from build123d import *

# Parameters (mm, degrees)
SKETCH_1_R          = 5.6
EXTRUDE_1_DEPTH     = 10
SKETCH_9_R          = 2.5
CUT_EXTRUDE_1_DEPTH = 6
SKETCH_11_R         = 2.5
CUT_EXTRUDE_2_DEPTH = 12


with BuildPart() as part:
    # 草图1 → 凸台-拉伸1 (new body)
    with BuildSketch(Plane.XY):
        with BuildLine():
            Line((-9.061643836, 9.77739726), (6.938356164, 9.77739726))
            ThreePointArc((6.938356164, 9.77739726), (8.352569727, 9.191610823), (8.938356164, 7.77739726))
            Line((8.938356164, 7.77739726), (8.938356164, -17.22260274))
            Line((8.938356164, -17.22260274), (-11.061643836, -17.22260274))
            Line((-11.061643836, -17.22260274), (-11.061643836, 7.77739726))
            ThreePointArc((-11.061643836, 7.77739726), (-10.475857398, 9.191610823), (-9.061643836, 9.77739726))
        make_face()
        with Locations((-1.061643836, -0.22260274)):
            Circle(SKETCH_1_R, mode=Mode.SUBTRACT)
    extrude(amount=EXTRUDE_1_DEPTH)

    # 草图9 → 切除-拉伸1 (cut)
    with BuildSketch(Plane(origin=(0, 9.77739726, 0), x_dir=(1, 0, 0), z_dir=(0, 1, 0))):
        with Locations((-1.061643836, -5)):
            Circle(SKETCH_9_R)
    extrude(amount=-CUT_EXTRUDE_1_DEPTH, mode=Mode.SUBTRACT)

    # 草图11 → 切除-拉伸2 (cut)
    with BuildSketch(Plane.XZ.offset(17.22260274)):
        with Locations((-6.061643836, 5)):
            Circle(SKETCH_11_R)
        with Locations((3.938356164, 5)):
            Circle(SKETCH_11_R)
    extrude(amount=-CUT_EXTRUDE_2_DEPTH, mode=Mode.SUBTRACT)


solid = part.part
CAD build for the part. Positions are in the model's coordinates, mm. A direction names the side the tool comes from. Round coordinates to 2 decimals unless told otherwise and drop trailing zeros. Write each loop counter-clockwise with the first axis right and the second up, starting at its lowest first coordinate (ties: lowest second). Pieces come first, ordered by that corner, then holes. Notation, with made-up numbers: (56, 23) -> (85, 23) arc R15 cw to (85, 35) -> close; hole circle Ø6 at (77, 65). An arc over 180 degrees is marked (long way). Answer as a JSON object with one key per item and string values.
(1) Band-saw the part on D-D, the plane x = 4. List the corners of the cut face in (y, z), then the cut area to 3 significant figures.
Reported:
{"outline": "(-17.22, 0) -> (-2.62, 0) -> (-2.62, 10) -> (-17.22, 10) -> (-17.22, 7.5) -> (-5.22, 7.5) -> (-5.22, 2.5) -> (-17.22, 2.5) -> close; (2.17, 0) -> (9.78, 0) -> (9.78, 10) -> (2.17, 10) -> close", "area": "162 mm^2"}
(2) Which spindle directions (+Z, -Z, +X, -X, +Y, -Y) get a long thin tool onto all of the face, cutting with end or side? Do faces 1 (the face through (-8.56, -11.31, 5.11)), 2 (the face through (-1, -17.223, 5)), 3 (the face through (-3.56, 7.32, 4.89)). Say none if no direction does.
Reported:
{"face 1": "-Y", "face 2": "+Z, -Z, +X, -X, -Y", "face 3": "+Y"}
(3) Band-saw the part on C-C, the plane y = -13. List the corners of the cut face in (x, z), then the cut area to 3 significant figures.
Reported:
{"outline": "(-11.06, 0) -> (8.94, 0) -> (8.94, 10) -> (-11.06, 10) -> close; hole circle Ø5 at (-6.06, 5); hole circle Ø5 at (3.94, 5)", "area": "161 mm^2"}
(4) Band-saw the part on A-A, the plane y = -4. List the corners of the cut face in (x, z), then the cut area to 3 significant figures.
Reported:
{"outline": "(-11.06, 0) -> (-5.2, 0) -> (-5.2, 10) -> (-11.06, 10) -> close; (3.07, 0) -> (8.94, 0) -> (8.94, 10) -> (3.07, 10) -> close", "area": "117 mm^2"}
(5) Probe probe 1 along X at (y, z) = (-7.75, 5); probe 2 along X at (y, z) = (0, 3.25); probe 3 along Z at (x, y) = (4, -11). List the from-to ranges inside material, lowest first. Write a range as [from, to].
Reported:
{"probe 1": "x = [-11.06, -8.56], [-3.56, 1.44], [6.44, 8.94]", "probe 2": "x = [-11.06, -6.66], [4.53, 8.94]", "probe 3": "z = [0, 2.5], [7.5, 10]"}
(6) Two-plate mould, pull along Y, no slides. Class faces 4 (the face through (-2.28, -5.69, 4.93)), 5 (the face through (8.938, -5, 5)), 6 (the face through (-3, 9.777, 3)): +Y half, -Y half, draft (parallel to the pull), parting line (faces both ways), or undercut.
Reported:
{"face 4": "undercut", "face 5": "draft", "face 6": "+Y half"}
(7) Pin check, flat tips, straight feed: P1, Ø4, axis at x = -1.06, z = 5, coming from the +Y side; P2, Ø2.5, axis at x = 4.5, z = 5, coming from the -Y side. Stop position of each tip, or through.
Reported:
{"P1": "stops at y = -5.45", "P2": "stops at y = -5.22"}
(8) Band-saw the part on B-B, the plane z = 5. List the corners of the cut face in (x, y).
Reported:
{"outline": "(-11.06, -17.22) -> (-8.56, -17.22) -> (-8.56, -5.22) -> (-3.58, -5.22) arc R5.6 cw to (-3.56, 4.79) -> (-3.56, 9.78) -> (-9.06, 9.78) arc R2 ccw to (-11.06, 7.78) -> close; (-3.56, -17.22) -> (1.44, -17.22) -> (1.44, -5.23) arc R5.6 cw to (-3.56, -5.23) -> close; (1.44, 4.79) arc R5.6 cw to (1.46, -5.22) -> (6.44, -5.22) -> (6.44, -17.22) -> (8.94, -17.22) -> (8.94, 7.78) arc R2 ccw to (6.94, 9.78) -> (1.44, 9.78) -> close"}
